```python
from build123d import *

# Parameters (mm, degrees)
SKETCH_1_W          = 50
SKETCH_1_H          = 30
EXTRUDE_1_DEPTH     = 84
SKETCH_2_W          = 26
SKETCH_2_H          = 14
CUT_EXTRUDE_1_DEPTH = 72
SKETCH_5_W          = 12
SKETCH_5_H          = 8
CUT_EXTRUDE_4_DEPTH = 94.407708461
SKETCH_6_W          = 12
SKETCH_6_H          = 8
CUT_EXTRUDE_5_DEPTH = 94.407708461
SKETCH_7_R          = 1.75
CUT_EXTRUDE_6_DEPTH = 93.633687177


with BuildPart() as part:
    # ｽｹｯﾁ1 → ﾎﾞｽ - 押し出し1 (new body)
    with BuildSketch(Plane.XY):
        Rectangle(SKETCH_1_W, SKETCH_1_H)
    extrude(amount=EXTRUDE_1_DEPTH)

    # ｽｹｯﾁ2 → ｶｯﾄ - 押し出し1 (cut)
    with BuildSketch(Plane(origin=(0, 0, 0), x_dir=(-1, 0, 0), z_dir=(0, 0, -1))):
        Rectangle(SKETCH_2_W, SKETCH_2_H)
    extrude(amount=-CUT_EXTRUDE_1_DEPTH, mode=Mode.SUBTRACT)

    # ｽｹｯﾁ5 → ｶｯﾄ - 押し出し4 (cut, through all)
    with BuildSketch(Plane.ZY.offset(-13)):
        with Locations((6, 0)):
            Rectangle(SKETCH_5_W, SKETCH_5_H)
    extrude(amount=-CUT_EXTRUDE_4_DEPTH, mode=Mode.SUBTRACT)

    # ｽｹｯﾁ6 → ｶｯﾄ - 押し出し5 (cut, through all)
    with BuildSketch(Plane(origin=(-13, 0, 0), x_dir=(0, 0, -1), z_dir=(1, 0, 0))):
        with Locations((-6, 0)):
            Rectangle(SKETCH_6_W, SKETCH_6_H)
    extrude(amount=-CUT_EXTRUDE_5_DEPTH, mode=Mode.SUBTRACT)

    # ｽｹｯﾁ7 → ｶｯﾄ - 押し出し6 (cut, through all)
    with BuildSketch(Plane(origin=(0, 15, 0), x_dir=(1, 0, 0), z_dir=(0, 1, 0))):
        with Locations(Location((19, -20, 0), (0, 0, 270))):
            Circle(SKETCH_7_R)
        with Locations(Location((19, -49, 0), (0, 0, 270))):
            Circle(SKETCH_7_R)
        with Locations(Location((19, -78, 0), (0, 0, 270))):
            Circle(SKETCH_7_R)
        with Locations(Location((0, -78, 0), (0, 0, 270))):
            Circle(SKETCH_7_R)
        with Locations(Location((-19, -78, 0), (0, 0, 270))):
            Circle(SKETCH_7_R)
        with Locations(Location((-19, -49, 0), (0, 0, 270))):
            Circle(SKETCH_7_R)
        with Locations(Location((-19, -20, 0), (0, 0, 270))):
            Circle(SKETCH_7_R)
    extrude(amount=-CUT_EXTRUDE_6_DEPTH, mode=Mode.SUBTRACT)

    # Surface Cut 1
    split(bisect_by=Plane(origin=(0, 0, 0), x_dir=(-1, 0, 0), z_dir=(0, -1, 0)), keep=Keep.TOP)


solid = part.part
```
For this review, take the finished solid that the model builds, in its own axes (mm). A direction names the side the tool comes from. Coordinates: 2 decimals unless noted, no trailing zeros. Write each loop counter-clockwise with the first axis right and the second up, starting at its lowest first coordinate (ties: lowest second). Pieces come first, ordered by that corner, then holes.
(1) Wall thickness on probe 1 along X at (y, z) = (-9.75, 20); probe 2 along X at (y, z) = (-3.5, 49); probe 3 along X at (y, z) = (-4.5, 78): over which ranges is each line inside the solid? List them lowest first.
(2) Add section B-B on z = 78. Give the boundary of the cut face in (x, y), then the cut area to 4 significant figures.
(3) Add section A-A on x = 19. Give the boundary of the cut face in (y, z), then the cut area to 3 significant figures.
(4) Add section C-C on y = -3. Give the boundary of the cut face in (x, z).
(5) Add section D-D on z = 49. Give the boundary of the cut face in (x, y).
(6) The part is to be moulded in two halves that separate along Z. For faces 4 (the face through (0, -7, 84)), 5 (the face through (19.526, -7.395, 50.669)), 6 (the face through (-19, -4, 6)), say which applies: +Z half, -Z half, draft (parallel to the pull), parting line (faces both ways), or undercut.
(7) For pin 1 Ø5.5 at (x, y) = (6, -2.5) entering from -Z; pin 2 Ø3 at (x, y) = (-17.5, -1) entering from -Z; pin 3 Ø6 at (x, z) = (-5.5, 60) entering from +Y, all flat-tipped, find the tip position at first contact; note any pin that passes through.
(8) Tool access review of faces 1 (the face through (-18.474, -7.395, 50.669)), 2 (the face through (0, -7, 35)), 3 (the face through (19, -2, 12)): name each direction out of +Z, -Z, +X, -X, +Y, -Y from which nothing blocks a thin tool from reaching the whole face with its end or side.
Answer sheet:
1. probe 1: x = -25 to -20.75, -17.25 to 17.25, 20.75 to 25
1. probe 2: x = -25 to -20.75, -17.25 to -13, 13 to 17.25, 20.75 to 25
1. probe 3: x = -25 to -20.75, -17.25 to -1.75, 1.75 to 17.25, 20.75 to 25
2. outline: (-25, -15) - (-20.75, -15) - (-20.75, 0) - (-25, 0) - close; (-17.25, -15) - (-1.75, -15) - (-1.75, 0) - (-17.25, 0) - close; (1.75, -15) - (17.25, -15) - (17.25, 0) - (1.75, 0) - close; (20.75, -15) - (25, -15) - (25, 0) - (20.75, 0) - close
2. area: 592.5 mm2
3. outline: (-15, 0) - (-4, 0) - (-4, 12) - (0, 12) - (0, 18.25) - (-15, 18.25) - close; (-15, 21.75) - (0, 21.75) - (0, 47.25) - (-15, 47.25) - close; (-15, 50.75) - (0, 50.75) - (0, 76.25) - (-15, 76.25) - close; (-15, 79.75) - (0, 79.75) - (0, 84) - (-15, 84) - close
3. area: 1,050 mm2
4. outline: (-25, 12) - (-13, 12) - (-13, 72) - (13, 72) - (13, 12) - (25, 12) - (25, 84) - (-25, 84) - close; hole circle Ø3.5 at (-19, 20); hole circle Ø3.5 at (-19, 49); hole circle Ø3.5 at (-19, 78); hole circle Ø3.5 at (0, 78); hole circle Ø3.5 at (19, 20); hole circle Ø3.5 at (19, 49); hole circle Ø3.5 at (19, 78)
5. outline: (-25, -15) - (-20.75, -15) - (-20.75, 0) - (-25, 0) - close; (-17.25, -15) - (17.25, -15) - (17.25, 0) - (13, 0) - (13, -7) - (-13, -7) - (-13, 0) - (-17.25, 0) - close; (20.75, -15) - (25, -15) - (25, 0) - (20.75, 0) - close
6. face 4: +Z half
6. face 5: undercut
6. face 6: draft
7. pin 1: stops at z = 72
7. pin 2: stops at z = 12
7. pin 3: stops at y = -7
8. face 1: +Y, -Y
8. face 2: -Z, +Y
8. face 3: -Z, +X, -X, +Y
